Read the model definition and answer for the solid it produces. Units are mm, in the model's axes. A direction names the side the tool comes from. Give positions to 0.01 mm unless a question says otherwise; leave off trailing zeros. Order: outer loops, then holes, each group sorted by start corner. A loop starts at its lowest first (then second) coordinate and runs counter-clockwise, first axis right, second up. Notation, with made-up numbers: (5.5, -19.75) - (10.5, -19.75) arc R20 ccw to (10.5, 5.25) - close; hole circle Ø7 at (57.5, 83). An arc over 180 degrees is marked (long way). Use a Markdown table: item, result. Add a question column.
1. Flat-ended cylindrical pins translate along their axes: P1, Ø10, axis at x = -0.5, z = 4, coming from the -Y side; P2, Ø3, axis at x = -0.5, z = -6.5, coming from the -Y side; P3, Ø5.5, axis at y = 6.5, z = -8.5, coming from the -X side; P4, Ø2, axis at x = 1, y = -1, coming from the -Z side. Find the tip coordinate at first contact, or state that the pin passes through.
2. Consider L1, parallel to Y at x = 0, z = -4.25; L2, parallel to X at y = 4, z = -8.75; L3, parallel to X at y = 0, z = -4.25. Determine where each line is inside the solid, lowest interval first.
3. Which of the six approach directions +Z, -Z, +X, -X, +Y, -Y give full straight-line access (tool end or side, diameter ignored) to faces 4 (the flat face through (0, 0, -2)), 5 (the cylindrical face through (9.715, 12.958, 1.699)), 6 (the flat face through (-4, 0, -3)), 7 (the cylindrical face through (5.699, -9.715, -7.288))?
4. For a pull along Z with two mould halves and no side action, classify faces 1 (the flat face through (6, 0, -1)), 2 (the flat face through (5, 0, -4.5)), 3 (the cylindrical face through (-9.715, 13.042, 1.699)) as released by +Z, released by -Z, zero draft, split by the parting line, or undercut.
5. A cutting plane is placed at B-B on z = -7. Determine the outline of the cut face in (x, y).
```python
from build123d import *

# Parameters (mm, degrees)
F0_W      = 20
F0_H      = 42
F1_DEPTH  = 2
F2_W      = 12
F2_H      = 20
F3_DEPTH  = 10
F4_R      = 1
F5_W      = 20
F5_H      = 10
F6_DEPTH  = 10
F7_R      = 4.99999
F8_R      = 3.6
F9_DEPTH  = 8
F10_W     = 2
F10_H     = 5
F11_DEPTH = 7
F12_R     = 5
F13_W     = 25
F13_H     = 2
F14_DEPTH = 2
F15_W     = 28.3062260176
F15_H     = 2
F16_DEPTH = 2
F17_R     = 1


# Not quite as in the source:
# - a fillet or chamfer is up to 0.001 mm smaller than in the source, because OpenCascade refuses the exact size


with BuildPart() as f1:
    # F0 (on Top) → F1 (new body)
    with BuildSketch(Plane.XY):
        Rectangle(F0_W, F0_H)
    extrude(amount=F1_DEPTH)

    # F2 (on Top) → F3 (join)
    with BuildSketch(Plane.XY):
        Rectangle(F2_W, F2_H)
    extrude(amount=-F3_DEPTH)

    # F4
    f4_edges = [f1.edges().sort_by_distance(p)[0] for p in [
        (-6, -10, -5),
        (6, -10, -5),
        (-6, 10, -5),
        (6, 10, -5),
    ]]
    fillet(f4_edges, radius=F4_R)

    # F5 (on face) → F6 (join)
    with BuildSketch(Plane.XY.offset(2)):
        Rectangle(F5_W, F5_H)
    extrude(amount=F6_DEPTH)

    # F7 (radius 5 in the source; OpenCascade refuses exactly that, so slightly less here)
    f7_edges = [f1.edges().sort_by_distance(p)[0] for p in [
        (0, -5, 12),
        (0, 5, 12),
        (0, -5, 2),
        (0, 5, 2),
    ]]
    fillet(f7_edges, radius=F7_R)

    # F8 (on face) → F9 (cut)
    with BuildSketch(Plane(origin=(0, 0, -10), x_dir=(1, 0, 0), z_dir=(0, 0, -1))):
        Circle(F8_R)
    extrude(amount=-F9_DEPTH, mode=Mode.SUBTRACT)

    # F10 (on face) → F11 (cut)
    with BuildSketch(Plane(origin=(0, 10, 0), x_dir=(-1, 0, 0), z_dir=(0, 1, 0))):
        with Locations((0, -7.5)):
            Rectangle(F10_W, F10_H)
    extrude(amount=-F11_DEPTH, mode=Mode.SUBTRACT)

    # F12
    f12_edges = [f1.edges().sort_by_distance(p)[0] for p in [
        (10, -21, 1),
        (-10, 21, 1),
        (10, 21, 1),
        (-10, -21, 1),
    ]]
    fillet(f12_edges, radius=F12_R)

    # F13 (on face) → F14 (cut)
    with BuildSketch(Plane(origin=(-6, 0, 0), x_dir=(0, -1, 0), z_dir=(-1, 0, 0))):
        with Locations((-0.9450479232, -3.5)):
            Rectangle(F13_W, F13_H)
    extrude(amount=-F14_DEPTH, mode=Mode.SUBTRACT)

    # F15 (on face) → F16 (cut)
    with BuildSketch(Plane.YZ.offset(6)):
        with Locations((-0.2904124558, -3.5)):
            Rectangle(F15_W, F15_H)
    extrude(amount=-F16_DEPTH, mode=Mode.SUBTRACT)

    # F17
    f17_edges = [f1.edges().sort_by_distance(p)[0] for p in [
        (-10, -3.535537, 10.535537),
    ]]
    fillet(f17_edges, radius=F17_R)


solid = f1.part
```
Output values:
| question | item | result |
|---|---|---|
| 1 | P1 | y = -21 |
| 1 | P2 | y = -10 |
| 1 | P3 | x = -6 |
| 1 | P4 | z = -2 |
| 2 | L1 | -10 to -3.6, 3.6 to 10 |
| 2 | L2 | -6 to -1, 1 to 6 |
| 2 | L3 | -4 to -3.6, 3.6 to 4 |
| 3 | face 4 | -Z |
| 3 | face 5 | +Z, +X, +Y |
| 3 | face 6 | -X, +Y, -Y |
| 3 | face 7 | -Z, +X, -Y |
| 4 | face 1 | zero draft |
| 4 | face 2 | undercut |
| 4 | face 3 | released by +Z |
| 5 | outline | (-6, -9) arc R1 ccw to (-5, -10) - (5, -10) arc R1 ccw to (6, -9) - (6, 9) arc R1 ccw to (5, 10) - (1, 10) - (1, 3.46) arc R3.6 cw (long way) to (-1, 3.46) - (-1, 10) - (-5, 10) arc R1 ccw to (-6, 9) - close |
